```python
from build123d import *

# Parameters (mm, degrees)
SKETCH_1_W              = 200
SKETCH_1_H              = 200
EXTRUDE_1_DEPTH         = 3
SKETCH_2_R              = 1.5
CUT_EXTRUDE_2_DEPTH     = 10
CUT_EXTRUDE_3_DEPTH     = 10
SKETCH_6_R              = 1.55
CUT_EXTRUDE_3_1_1_DEPTH = 10
CUT_EXTRUDE_6_REACH     = 111.495
SKETCH_11_R             = 1.5
CUT_EXTRUDE_20_5_REACH  = 111.495
SKETCH_4_R              = 11.25
FILLET_1_R              = 1
SKETCH_12_W             = 40
SKETCH_12_H             = 3
EXTRUDE_2_DEPTH         = 75
FILLET_2_R              = 7
SKETCH_13_R             = 1.55
CUT_EXTRUDE_3_1_3_DEPTH = 10
CUT_EXTRUDE_2006_REACH  = 132.367
SKETCH_14_R             = 1.55
SKETCH_14_R_2           = 6.6
FILLET_3_R              = 8
SKETCH_17_R             = 1.55
CUT_EXTRUDE_7_DEPTH     = 131.36679025


with BuildPart() as part:
    # 草图1 → 凸台-拉伸1 (new body)
    with BuildSketch(Plane(origin=(0, 0, 0), x_dir=(1, 0, 0), z_dir=(0, 1, 0))):
        Rectangle(SKETCH_1_W, SKETCH_1_H)
    extrude(amount=EXTRUDE_1_DEPTH)

    # 草图2 → 切除-拉伸2 (cut)
    with BuildSketch(Plane(origin=(0, 3, 0), x_dir=(1, 0, 0), z_dir=(0, 1, 0))):
        with Locations(Location((29.5, 9.5, 0), (0, 0, 270))):
            Circle(SKETCH_2_R)
        with Locations(Location((21.5, 0, 0), (0, 0, 270))):
            Circle(SKETCH_2_R)
        with Locations(Location((29.5, -9.5, 0), (0, 0, 270))):
            Circle(SKETCH_2_R)
        with Locations(Location((37.5, 0, 0), (0, 0, 270))):
            Circle(SKETCH_2_R)
        with Locations(Location((-29.5, -9.5, 0), (0, 0, 270))):
            Circle(SKETCH_2_R)
        with Locations(Location((-37.5, 0, 0), (0, 0, 270))):
            Circle(SKETCH_2_R)
        with Locations(Location((-21.5, 0, 0), (0, 0, 270))):
            Circle(SKETCH_2_R)
        with Locations(Location((-29.5, 9.5, 0), (0, 0, 270))):
            Circle(SKETCH_2_R)
    extrude(amount=-CUT_EXTRUDE_2_DEPTH, mode=Mode.SUBTRACT)

    # 草图5 → 切除-拉伸3 (cut)
    with BuildSketch(Plane(origin=(0, 3, 0), x_dir=(1, 0, 0), z_dir=(0, 1, 0))):
        with BuildLine():
            Line((-100, -100), (-44.5, -100))
            Line((-44.5, -100), (-44.5, 0))
            ThreePointArc((-44.5, 0), (-40.212142643, 10.5), (-29.8, 14.9969997))
            ThreePointArc((-29.8, 14.9969997), (-22.858571571, 17.9949995), (-20, 24.9949995))
            Line((-20, 24.9949995), (-20, 47.5))
            Line((-20, 47.5), (0, 47.5))
            Line((0, 47.5), (20, 47.5))
            Line((20, 47.5), (20, 24.9949995))
            ThreePointArc((20, 24.9949995), (22.858571571, 17.9949995), (29.8, 14.9969997))
            ThreePointArc((29.8, 14.9969997), (40.212142643, 10.5), (44.5, 0))
            Line((44.5, 0), (44.5, -100))
            Line((44.5, -100), (100, -100))
            Line((100, -100), (100, 100))
            Line((100, 100), (-100, 100))
            Line((-100, 100), (-100, -100))
        make_face()
    extrude(amount=-CUT_EXTRUDE_3_DEPTH, mode=Mode.SUBTRACT)

    # 草图6 → φ3.1通孔1 (cut)
    with BuildSketch(Plane.XZ):
        with Locations(Location((-15, -42.5, 0), (0, 0, 270))):
            Circle(SKETCH_6_R)
        with Locations(Location((-15, -27.5, 0), (0, 0, 270))):
            Circle(SKETCH_6_R)
        with Locations(Location((15, -27.5, 0), (0, 0, 90))):
            Circle(SKETCH_6_R)
        with Locations(Location((15, -42.5, 0), (0, 0, 90))):
            Circle(SKETCH_6_R)
    extrude(amount=-CUT_EXTRUDE_3_1_1_DEPTH, mode=Mode.SUBTRACT)

    # 草图11 → 切除-拉伸6 (cut, up to next)
    with BuildSketch(Plane(origin=(0, 3, 0), x_dir=(1, 0, 0), z_dir=(0, 1, 0)), mode=Mode.PRIVATE) as cut_extrude_6_sk1:
        with BuildLine():
            Line((44.5, -17.5), (44.5, -100))
            Line((44.5, -100), (101.133062566, -100))
            Line((101.133062566, -100), (101.133062566, 47.5))
            Line((101.133062566, 47.5), (20, 47.5))
            Line((20, 47.5), (20, 7.5))
            Line((20, 7.5), (19, 7.5))
            ThreePointArc((19, 7.5), (18.292893219, 7.207106781), (18, 6.5))
            Line((18, 6.5), (18, -4))
            ThreePointArc((18, -4), (20.48959236, -10.01040764), (26.5, -12.5))
            Line((26.5, -12.5), (39.5, -12.5))
            Line((39.5, -12.5), (44.5, -12.5))
            Line((44.5, -12.5), (44.5, -17.5))
        make_face()
        with Locations((29.5, -9.5)):
            Circle(SKETCH_11_R, mode=Mode.SUBTRACT)
        with Locations((21.5, 0)):
            Circle(SKETCH_11_R, mode=Mode.SUBTRACT)
    cut_extrude_6_tool1 = extrude(cut_extrude_6_sk1.sketch, amount=-CUT_EXTRUDE_6_REACH, mode=Mode.PRIVATE) & part.part
    # 草图11 → 切除-拉伸6 (cut, up to next)
    with BuildSketch(Plane(origin=(0, 3, 0), x_dir=(1, 0, 0), z_dir=(0, 1, 0)), mode=Mode.PRIVATE) as cut_extrude_6_sk2:
        with BuildLine():
            Line((-44.5, -17.5), (-44.5, -100))
            Line((-44.5, -100), (-101.133062566, -100))
            Line((-101.133062566, -100), (-101.133062566, 47.5))
            Line((-101.133062566, 47.5), (-20, 47.5))
            Line((-20, 47.5), (-20, 7.5))
            Line((-20, 7.5), (-19, 7.5))
            ThreePointArc((-19, 7.5), (-18.292893219, 7.207106781), (-18, 6.5))
            Line((-18, 6.5), (-18, -4))
            ThreePointArc((-18, -4), (-20.48959236, -10.01040764), (-26.5, -12.5))
            Line((-26.5, -12.5), (-39.5, -12.5))
            Line((-39.5, -12.5), (-44.5, -12.5))
            Line((-44.5, -12.5), (-44.5, -17.5))
        make_face()
    cut_extrude_6_tool2 = extrude(cut_extrude_6_sk2.sketch, amount=-CUT_EXTRUDE_6_REACH, mode=Mode.PRIVATE) & part.part
    add(cut_extrude_6_tool1.solids().sort_by_distance((66.686037, 3, 19.669577))[0], mode=Mode.SUBTRACT)
    add(cut_extrude_6_tool2.solids().sort_by_distance((-66.626911, 3, 19.648158))[0], mode=Mode.SUBTRACT)

    # 草图4 → φ20.5落弹孔 (cut, up to next)
    with BuildSketch(Plane(origin=(0, 3, 0), x_dir=(1, 0, 0), z_dir=(0, 1, 0)), mode=Mode.PRIVATE) as cut_extrude_20_5_sk1:
        with Locations(Location((0, -29, 0), (0, 0, 270))):
            Circle(SKETCH_4_R)
    cut_extrude_20_5_tool1 = extrude(cut_extrude_20_5_sk1.sketch, amount=-CUT_EXTRUDE_20_5_REACH, mode=Mode.PRIVATE) & part.part
    add(cut_extrude_20_5_tool1.solids().sort_by_distance((0, 3, 29))[0], mode=Mode.SUBTRACT)

    # 圆角1
    fillet_1_edges = [part.edges().sort_by_distance(p)[0] for p in [
        (-20, 1.5, -7.5),
        (20, 1.5, -7.5),
    ]]
    fillet(fillet_1_edges, radius=FILLET_1_R - 0.0001)  # a hair under: the kernel refuses the full size

    # 草图12 → 凸台-拉伸2 (add)
    with BuildSketch(Plane(origin=(0, 0, -47.5), x_dir=(-1, 0, 0), z_dir=(0, 0, -1))):
        with Locations((0, 1.5)):
            Rectangle(SKETCH_12_W, SKETCH_12_H)
    extrude(amount=EXTRUDE_2_DEPTH)

    # 圆角2
    fillet_2_edges = [part.edges().sort_by_distance(p)[0] for p in [
        (20, 1.5, -122.5),
        (-20, 1.5, -122.5),
    ]]
    fillet(fillet_2_edges, radius=FILLET_2_R)

    # 草图13 → φ3.1通孔3 (cut)
    with BuildSketch(Plane(origin=(0, 3, 0), x_dir=(1, 0, 0), z_dir=(0, 1, 0))):
        with Locations(Location((-8.625, 113.5, 0), (0, 0, 270))):
            Circle(SKETCH_13_R)
        with Locations(Location((8.625, 113.5, 0), (0, 0, 270))):
            Circle(SKETCH_13_R)
        with Locations(Location((8.625, 73.5, 0), (0, 0, 270))):
            Circle(SKETCH_13_R)
        with Locations(Location((-8.625, 73.5, 0), (0, 0, 270))):
            Circle(SKETCH_13_R)
    extrude(amount=-CUT_EXTRUDE_3_1_3_DEPTH, mode=Mode.SUBTRACT)

    # 草图14 → 2006电机固定 (cut, up to next)
    with BuildSketch(Plane(origin=(0, 3, 0), x_dir=(1, 0, 0), z_dir=(0, 1, 0)), mode=Mode.PRIVATE) as cut_extrude_2006_sk1:
        with Locations(Location((0, -63.5, 0), (0, 0, 270))):
            Circle(SKETCH_14_R)
    cut_extrude_2006_tool1 = extrude(cut_extrude_2006_sk1.sketch, amount=-CUT_EXTRUDE_2006_REACH, mode=Mode.PRIVATE) & part.part
    # 草图14 → 2006电机固定 (cut, up to next)
    with BuildSketch(Plane(origin=(0, 3, 0), x_dir=(1, 0, 0), z_dir=(0, 1, 0)), mode=Mode.PRIVATE) as cut_extrude_2006_sk2:
        with Locations(Location((-8.227241336, -49.25, 0), (0, 0, 270))):
            Circle(SKETCH_14_R)
    cut_extrude_2006_tool2 = extrude(cut_extrude_2006_sk2.sketch, amount=-CUT_EXTRUDE_2006_REACH, mode=Mode.PRIVATE) & part.part
    # 草图14 → 2006电机固定 (cut, up to next)
    with BuildSketch(Plane(origin=(0, 3, 0), x_dir=(1, 0, 0), z_dir=(0, 1, 0)), mode=Mode.PRIVATE) as cut_extrude_2006_sk3:
        with Locations(Location((8.227241336, -49.25, 0), (0, 0, 270))):
            Circle(SKETCH_14_R)
    cut_extrude_2006_tool3 = extrude(cut_extrude_2006_sk3.sketch, amount=-CUT_EXTRUDE_2006_REACH, mode=Mode.PRIVATE) & part.part
    # 草图14 → 2006电机固定 (cut, up to next)
    with BuildSketch(Plane(origin=(0, 3, 0), x_dir=(1, 0, 0), z_dir=(0, 1, 0)), mode=Mode.PRIVATE) as cut_extrude_2006_sk4:
        with Locations(Location((0, -54, 0), (0, 0, 270))):
            Circle(SKETCH_14_R_2)
    cut_extrude_2006_tool4 = extrude(cut_extrude_2006_sk4.sketch, amount=-CUT_EXTRUDE_2006_REACH, mode=Mode.PRIVATE) & part.part
    add(cut_extrude_2006_tool1.solids().sort_by_distance((0, 3, 63.5))[0], mode=Mode.SUBTRACT)
    add(cut_extrude_2006_tool2.solids().sort_by_distance((-8.227241, 3, 49.25))[0], mode=Mode.SUBTRACT)
    add(cut_extrude_2006_tool3.solids().sort_by_distance((8.227241, 3, 49.25))[0], mode=Mode.SUBTRACT)
    add(cut_extrude_2006_tool4.solids().sort_by_distance((0, 3, 54))[0], mode=Mode.SUBTRACT)

    # 圆角3
    fillet_3_edges = [part.edges().sort_by_distance(p)[0] for p in [
        (44.5, 1.5, 12.5),
        (-44.5, 1.5, 12.5),
    ]]
    fillet(fillet_3_edges, radius=FILLET_3_R)

    # 草图17 → 切除-拉伸7 (cut, through all)
    with BuildSketch(Plane(origin=(0, 3, 0), x_dir=(1, 0, 0), z_dir=(0, 1, 0))):
        with Locations(Location((-40.5, -30, 0), (0, 0, 270))):
            Circle(SKETCH_17_R)
        with Locations(Location((-40.5, -52, 0), (0, 0, 270))):
            Circle(SKETCH_17_R)
    cut_extrude_7 = extrude(amount=-CUT_EXTRUDE_7_DEPTH, mode=Mode.SUBTRACT)

    # 镜向1: 切除-拉伸7 across plane
    add(cut_extrude_7.mirror(Plane(origin=(0, 0, 0), x_dir=(0, 0, 1), z_dir=(1, 0, 0))), mode=Mode.SUBTRACT)


solid = part.part
```
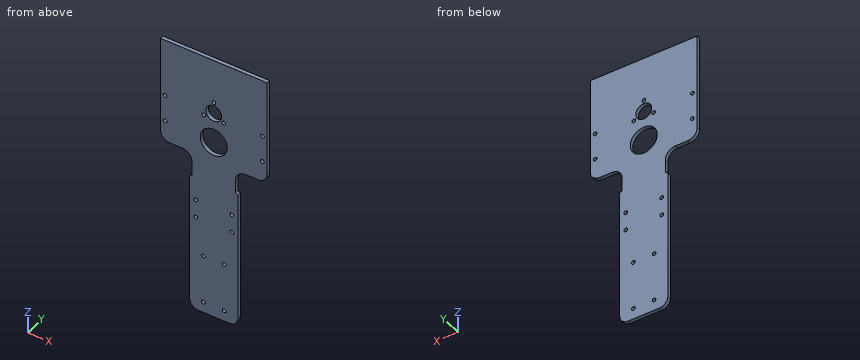
Part model, mm, in its own coordinate system. Round coordinates to 2 decimals unless told otherwise and drop trailing zeros. Loops run counter-clockwise (first coordinate to the right, second up) from the corner with the lowest first, then second, coordinate; pieces in that order, holes last.
Item 1: Drop a flat-ended pin along its axis: P1, Ø0.9, axis at y = 1, z = -2.5, coming from the -X side. Give the stop position or say it passes through.
Item 2: Cut at C-C, the plane y = 1.95. State how many separate pieces and enclosed holes the cut face has, then the cut area to 3 significant figures.
Item 3: Cut at B-B, the plane x = -34.5. Give the cut face in (y, z).
Item 4: Drill centre lines: line 1 (X direction, y = 1.9, z = -73.5) (3 decimals); line 2 (X direction, y = 2.35, z = -42.5); line 3 (Z direction, x = 3, y = 0.25). Where is each one in solid material? Low to high.
Item 5: Cut at A-A, the plane z = 36. Give the cut face in (x, y), then the cut area to 3 significant figures.
A:
1. P1: stops at x = -18
2. separate pieces: 1
2. enclosed holes: 17
2. area: 12,400 mm2
3. outline: (0, 12.5) - (3, 12.5) - (3, 100) - (0, 100) - close
4. line 1: x = -20 to -10.175, -7.075 to 7.075, 10.175 to 20
4. line 2: x = -20 to -16.55, -13.45 to 13.45, 16.55 to 20
4. line 3: z = -122.5 to 18.16, 39.84 to 48.12, 59.88 to 100
5. outline: (-44.5, 0) - (-8.81, 0) - (-8.81, 3) - (-44.5, 3) - close; (8.81, 0) - (44.5, 0) - (44.5, 3) - (8.81, 3) - close
5. area: 214 mm2
